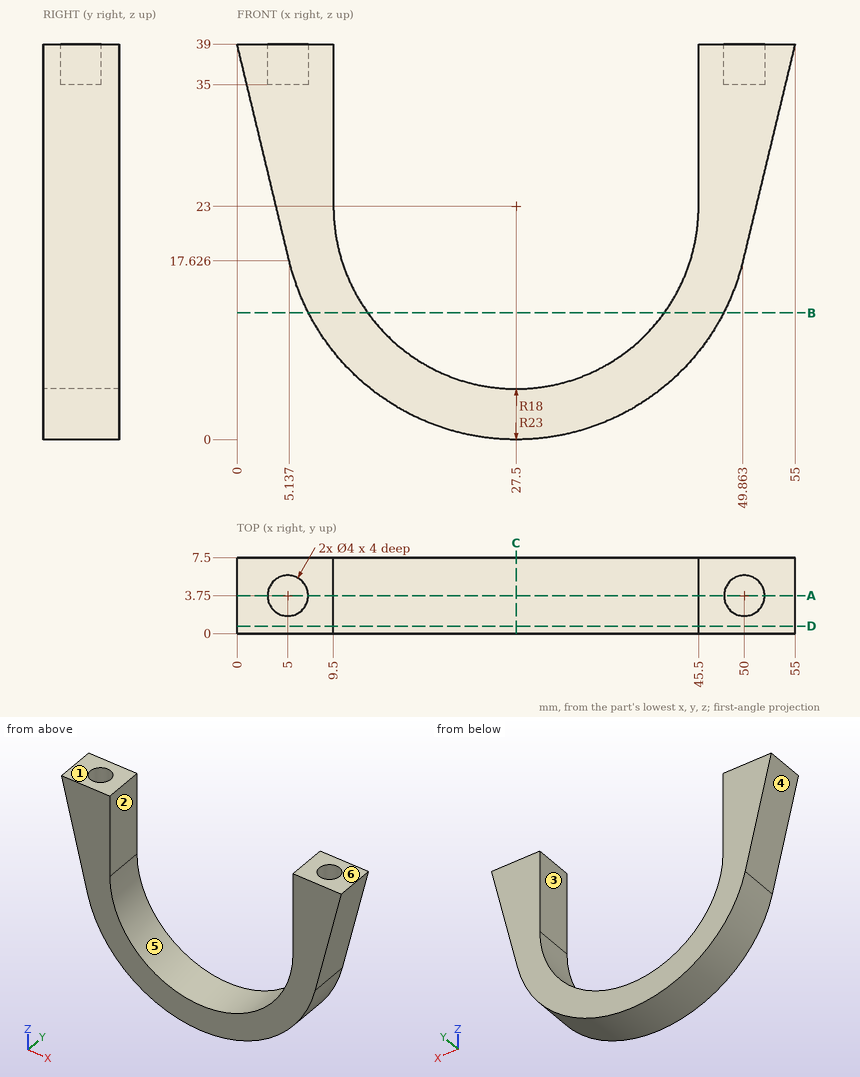
Geometry: see drawing. Coordinates: mm, zero at the bounding-box minimum. A direction names the side the tool comes from. Round coordinates to 2 decimals unless told otherwise and drop trailing zeros. Order: outer loops, then holes, each group sorted by start corner. A loop starts at its lowest first (then second) coordinate and runs counter-clockwise, first axis right, second up. Notation, with made-up numbers: (-37, 10) -> (14, 10) arc R29 cw to (14, 41) -> close; hole circle Ø5 at (18.25, 17.25). An arc over 180 degrees is marked (long way). Use CSV: the item, a comma, the result in double quotes.
(1) Access query for the marked faces 1 and 2. Directions: +Z, -Z, +X, -X, +Y, -Y. A direction counts if a zero-diameter tool reaches every point of the face in a straight line with its end or side. Return the directions, or none.
Report:
face 1,"+Z, +X, -X, +Y, -Y"
face 2,"+Z, +Y, -Y"
(2) Section A-A on y = 3.75. Return the cut outline in (x, z) (1 decimal).
Report:
outline,"(0, 39) -> (5.1, 17.6) arc R23 ccw to (49.9, 17.6) -> (55, 39) -> (52, 39) -> (52, 35) -> (48, 35) -> (48, 39) -> (45.5, 39) -> (45.5, 23) arc R18 cw to (9.5, 23) -> (9.5, 39) -> (7, 39) -> (7, 35) -> (3, 35) -> (3, 39) -> close"
(3) Pull-direction query (X, two-part tool) for the marked faces 3, 4, 5 and 6; classes: +X half, -X half, draft (parallel to the pull), parting line (faces both ways), or undercut.
Report:
face 3,"undercut"
face 4,"-X half"
face 5,"undercut"
face 6,"draft"
(4) Section B-B on z = 12.5. Return the cut outline in (x, y).
Report:
outline,"(7.04, 0) -> (12.88, 0) -> (12.88, 7.5) -> (7.04, 7.5) -> close; (42.12, 0) -> (47.96, 0) -> (47.96, 7.5) -> (42.12, 7.5) -> close"
(5) Section C-C on x = 27.5. Return the cut outline in (y, z).
Report:
outline,"(0, 0) -> (7.5, 0) -> (7.5, 5) -> (0, 5) -> close"
(6) Ray query, L1, parallel to Y at x = 50, z = 36.35; L2, parallel to X at y = 1.5, z = 29; L3, parallel to X at y = 2.25, z = 11 (1 decimal). Return the intervals inside material, ascending.
Report:
L1,"0 to 1.75, 5.75 to 7.5"
L2,"2.4 to 9.5, 45.5 to 52.6"
L3,"7.9 to 14.1, 40.9 to 47.1"
(7) First-contact query: pin 1 Ø12 at (x, z) = (35, 30) entering from +Y; pin 2 Ø2.5 at (x, y) = (5, 3.75) entering from +Z; pin 3 Ø8 at (x, z) = (31, 6) entering from -Y; pin 4 Ø1.5 at (x, y) = (30, 3.5) entering from -Z. Flat tips, straight axial feed; report the tip coordinate or a pass-through.
Report:
pin 1,"through"
pin 2,"z = 35"
pin 3,"y = 0"
pin 4,"z = 0.07"
(8) Section D-D on y = 0.75. Return the cut outline in (x, z) (1 decimal), and give its area (3 significant figures).
Report:
outline,"(0, 39) -> (5.1, 17.6) arc R23 ccw to (49.9, 17.6) -> (55, 39) -> (45.5, 39) -> (45.5, 23) arc R18 cw to (9.5, 23) -> (9.5, 39) -> close"
area,"567 mm^2"
